Part model, mm, in its own coordinate system. A direction names the side the tool comes from. Coordinates: 2 decimals unless noted, no trailing zeros. Loops run counter-clockwise (first coordinate to the right, second up) from the corner with the lowest first, then second, coordinate; pieces in that order, holes last. Notation, with made-up numbers: (-28.5, 3.25) - (1.5, 3.25) arc R24 cw to (1.5, 23.25) - close; hole circle Ø10 at (-27.5, 88). An arc over 180 degrees is marked (long way). Answer as CSV lines item,"result".
from build123d import *

# Parameters (mm, degrees)
SKETCH1_R               = 5
BOSS_EXTRUDE1_DEPTH     = 60
CUT_EXTRUDE2_DEPTH      = 61.415229868
CUT_EXTRUDE2_DEPTH_BACK = 61.415229868
SKETCH3_R               = 2.25
SKETCH4_R               = 5
SKETCH4_R_2             = 4.65
CUT_EXTRUDE3_DEPTH      = 1
CUT_EXTRUDE4_START      = 1
SKETCH5_R               = 5
SKETCH5_R_2             = 4.65
CUT_EXTRUDE4_DEPTH      = 1
CUT_EXTRUDE5_DEPTH      = 61.415229984
CUT_EXTRUDE5_DEPTH_BACK = 61.415229984
SKETCH6_R               = 2.5


with BuildPart() as part:
    # Sketch1 → Boss-Extrude1 (new, symmetric)
    with BuildSketch(Plane(origin=(0, 0, 0), x_dir=(1, 0, 0), z_dir=(0, 1, 0))):
        with Locations(Location((0, 0, 0), (0, 0, 270))):
            Circle(SKETCH1_R)
    extrude(amount=BOSS_EXTRUDE1_DEPTH, both=True)

    # Sketch3 → Cut-Extrude2 (cut, two sides: drawn at the far end of the back side and taken through both)
    with BuildSketch(Plane.XY.offset(-CUT_EXTRUDE2_DEPTH_BACK)):
        with Locations(Location((0, -35, 0), (0, 0, 89.999999993))):
            Circle(SKETCH3_R)
    extrude(amount=CUT_EXTRUDE2_DEPTH + CUT_EXTRUDE2_DEPTH_BACK, mode=Mode.SUBTRACT)

    # Sketch4 → Cut-Extrude3 (cut)
    with BuildSketch(Plane(origin=(0, -28, 0), x_dir=(-1, 0, 0), z_dir=(0, -1, 0))):
        with Locations(Location((0, 0, 0), (0, 0, 90))):
            Circle(SKETCH4_R)
        with Locations(Location((0, 0, 0), (0, 0, 90))):
            Circle(SKETCH4_R_2, mode=Mode.SUBTRACT)
    extrude(amount=CUT_EXTRUDE3_DEPTH, mode=Mode.SUBTRACT)

    # Sketch5 → Cut-Extrude4 (cut)
    with BuildSketch(Plane(origin=(0, 55, 0), x_dir=(1, 0, 0), z_dir=(0, 1, 0)).offset(CUT_EXTRUDE4_START)):
        with Locations(Location((0, 0, 0), (0, 0, 90))):
            Circle(SKETCH5_R)
        with Locations(Location((0, 0, 0), (0, 0, 90))):
            Circle(SKETCH5_R_2, mode=Mode.SUBTRACT)
    extrude(amount=-CUT_EXTRUDE4_DEPTH, mode=Mode.SUBTRACT)

    # Sketch6 → Cut-Extrude5 (cut, two sides: drawn at the far end of the back side and taken through both)
    with BuildSketch(Plane(origin=(0, 0, 0), x_dir=(0, 0, -1), z_dir=(1, 0, 0)).offset(-CUT_EXTRUDE5_DEPTH_BACK)):
        with Locations((0, 15)):
            Circle(SKETCH6_R)
    extrude(amount=CUT_EXTRUDE5_DEPTH + CUT_EXTRUDE5_DEPTH_BACK, mode=Mode.SUBTRACT)


solid = part.part
Q1. Saw through at D-D (y = -35). Give the cut face in (x, z).
Results:
outline,"(-2.25, -4.47) - (-2.25, 4.47) arc R5 ccw to start; (2.25, -4.47) arc R5 ccw to (2.25, 4.47) - close"
Q2. Saw through at B-B (x = -1). Give the cut face in (y, z).
Results:
outline,"(-60, -4.9) - (-37.02, -4.9) - (-37.02, 4.9) - (-60, 4.9) - close; (-32.98, -4.9) - (-29, -4.9) - (-29, -4.54) - (-28, -4.54) - (-28, -4.9) - (55, -4.9) - (55, -4.54) - (56, -4.54) - (56, -4.9) - (60, -4.9) - (60, 4.9) - (56, 4.9) - (56, 4.54) - (55, 4.54) - (55, 4.9) - (-28, 4.9) - (-28, 4.54) - (-29, 4.54) - (-29, 4.9) - (-32.98, 4.9) - close; hole circle Ø5 at (15, 0)"
Q3. Two-plate mould, pull along Z, no slides. Class faces 1 (the face through (0, 60, 0)), 2 (the face through (-0.07, 14.04, -2.31)), 3 (the face through (4, 14, 3)): released by +Z, released by -Z, zero draft, split by the parting line, or undercut.
Results:
face 1,"zero draft"
face 2,"undercut"
face 3,"split by the parting line"
Q4. Wall check: L1, parallel to Y at x = -0.25, z = 0; L2, parallel to Y at x = -1.5, z = 0; L3, parallel to Y at x = -4, z = 0. Give the ranges that are in metal, low to high.
Results:
L1,"y = -60 to -37.24, -32.76 to 12.5, 17.5 to 60"
L2,"y = -60 to -36.68, -33.32 to 12.5, 17.5 to 60"
L3,"y = -60 to 12.5, 17.5 to 60"
Q5. Flat gauge pins, fed straight in: pin 1 (3 mm diameter, centred on y = 14.5, z = 3.5, fed in from -X); pin 2 (5 mm diameter, centred on y = -9.5, z = 3.5, fed in from -X); pin 3 (4 mm diameter, centred on x = 0, y = -35, fed in from -Z); pin 4 (3 mm diameter, centred on y = -13.5, z = 3.5, fed in from -X). Where does each tip first touch, or does it go through?
Results:
pin 1,"stops at x = -4.5"
pin 2,"stops at x = -4.9"
pin 3,"passes through"
pin 4,"stops at x = -4.58"
Q6. Which spindle directions (+Z, -Z, +X, -X, +Y, -Y) get a long thin tool onto all of the face, cutting with end or side? Do faces 4 (the face through (-0.676, -32.854, -0.072)), 5 (the face through (1.397, -28.493, -4.435)). Say none if no direction does.
Results:
face 4,"+Z, -Z"
face 5,"none"
Q7. Saw through at C-C (x = 3.25). Give the cut face in (y, z).
Results:
outline,"(-60, -3.8) - (-29, -3.8) - (-29, -3.33) - (-28, -3.33) - (-28, -3.8) - (55, -3.8) - (55, -3.33) - (56, -3.33) - (56, -3.8) - (60, -3.8) - (60, 3.8) - (56, 3.8) - (56, 3.33) - (55, 3.33) - (55, 3.8) - (-28, 3.8) - (-28, 3.33) - (-29, 3.33) - (-29, 3.8) - (-60, 3.8) - close; hole circle Ø5 at (15, 0)"
Q8. Saw through at A-A (z = 0). Give the cut face in (x, y).
Results:
outline,"(-5, -60) - (5, -60) - (5, -29) - (4.65, -29) - (4.65, -28) - (5, -28) - (5, 12.5) - (-5, 12.5) - (-5, -28) - (-4.65, -28) - (-4.65, -29) - (-5, -29) - close; (-5, 17.5) - (5, 17.5) - (5, 55) - (4.65, 55) - (4.65, 56) - (5, 56) - (5, 60) - (-5, 60) - (-5, 56) - (-4.65, 56) - (-4.65, 55) - (-5, 55) - close; hole circle Ø4.5 at (0, -35)"
